Geometry: final body of the model. Coordinates: model frame, mm. Face numbers are marked on the shaded views. A direction names the side the tool comes from. Give positions to 0.01 mm unless a question says otherwise; leave off trailing zeros. Loops run counter-clockwise (first coordinate to the right, second up) from the corner with the lowest first, then second, coordinate; pieces in that order, holes last. Notation, with made-up numbers: (-9.75, 34.25) -> (30.25, 34.25) arc R19 cw to (30.25, 40.25) -> close; hole circle Ø11 at (31.25, 76.25). An arc over 180 degrees is marked (long way). Answer in a Markdown table with one row per item. Add a question column.
from build123d import *

# Parameters (mm, degrees)
SKETCH1_R               = 6
BOSS_EXTRUDE1_DEPTH     = 20
SKETCH2_R               = 2.25
CUT_EXTRUDE1_DEPTH      = 20
SKETCH4_R               = 1.5
CUT_EXTRUDE2_DEPTH      = 45
BOSS_EXTRUDE2_START     = 11
SKETCH5_W               = 15.288681569
SKETCH5_H               = 20
SKETCH5_R               = 1.5
BOSS_EXTRUDE2_DEPTH     = 11
CUT_EXTRUDE3_REACH      = 89.238
CUT_EXTRUDE3_END_RADIUS = 6
SKETCH6_R               = 1.25
SKETCH7_R               = 3
CUT_EXTRUDE4_DEPTH      = 5
CUT_EXTRUDE5_DEPTH      = 5
FILLET1_R               = 5
BOSS_EXTRUDE3_START     = 1
SKETCH10_R              = 3
SKETCH10_R_2            = 1.5
BOSS_EXTRUDE3_DEPTH     = 1
CHAMFER1_SIZE           = 1
SKETCH11_R              = 3
SKETCH11_R_2            = 1.5
BOSS_EXTRUDE4_DEPTH     = 1
CHAMFER2_SIZE           = 1


with BuildPart() as part:
    # Sketch1 → Boss-Extrude1 (new body)
    with BuildSketch(Plane.XY):
        Polygon((27, 30.8), (27, 25.8), (13, 25.8), (13, -7), (42, -7), (42, -13), (-7, -13), (-7, -43), (-13, -43), (-13, -8.291544952), (-13, 30.8), align=None)
        with Locations((0.051684878, 5)):
            Circle(SKETCH1_R, mode=Mode.SUBTRACT)
    extrude(amount=BOSS_EXTRUDE1_DEPTH)

    # Sketch2 → Cut-Extrude1 (cut)
    with BuildSketch(Plane.ZY.offset(13)):
        with Locations(Location((10, -38, 0), (0, 0, 270))):
            Circle(SKETCH2_R)
        with Locations(Location((10, -23, 0), (0, 0, 270))):
            Circle(SKETCH2_R)
    extrude(amount=-CUT_EXTRUDE1_DEPTH, mode=Mode.SUBTRACT)

    # Sketch4 → Cut-Extrude2 (cut)
    with BuildSketch(Plane(origin=(0, 30.8, 0), x_dir=(1, 0, 0), z_dir=(0, 1, 0))):
        with Locations(Location((22, -10, 0), (0, 0, 180))):
            Circle(SKETCH4_R)
        with Locations(Location((36, -10, 0), (0, 0, 180))):
            Circle(SKETCH4_R)
    extrude(amount=-CUT_EXTRUDE2_DEPTH, mode=Mode.SUBTRACT)

    # Sketch5 → Boss-Extrude2 (add)
    with BuildSketch(Plane(origin=(0, -7, 0), x_dir=(1, 0, 0), z_dir=(0, 1, 0)).offset(BOSS_EXTRUDE2_START)):
        with Locations((20.355659216, -10)):
            Rectangle(SKETCH5_W, SKETCH5_H)
        with Locations(Location((22, -10, 0), (0, 0, 180))):
            Circle(SKETCH5_R, mode=Mode.SUBTRACT)
    extrude(amount=-BOSS_EXTRUDE2_DEPTH)

    # Cut-Extrude3: up to this cylinder (the profile starts outside it)
    cut_extrude3_end = Plane(origin=(0.051684878, 5, 10), z_dir=(0, 0, -1)) * Cylinder(CUT_EXTRUDE3_END_RADIUS, 191.476, mode=Mode.PRIVATE)
    # Sketch6 → Cut-Extrude3 (cut, up to the surface)
    with BuildSketch(Plane(origin=(0, 30.8, 0), x_dir=(1, 0, 0), z_dir=(0, 1, 0)), mode=Mode.PRIVATE) as cut_extrude3_sk1:
        with Locations(Location((0, -10, 0), (0, 0, 180))):
            Circle(SKETCH6_R)
    cut_extrude3_tool1 = extrude(cut_extrude3_sk1.sketch, amount=-CUT_EXTRUDE3_REACH, mode=Mode.PRIVATE) - cut_extrude3_end
    add(cut_extrude3_tool1.solids().sort_by_distance((0, 30.8, 10))[0], mode=Mode.SUBTRACT)

    # Sketch7 → Cut-Extrude4 (cut)
    with BuildSketch(Plane(origin=(0, 30.8, 0), x_dir=(1, 0, 0), z_dir=(0, 1, 0))):
        with Locations(Location((0, -10, 0), (0, 0, 180))):
            Circle(SKETCH7_R)
    extrude(amount=-CUT_EXTRUDE4_DEPTH, mode=Mode.SUBTRACT)

    # Sketch9 → Cut-Extrude5 (cut)
    with BuildSketch(Plane.XZ.offset(13)):
        Polygon((25.233161507, 10), (23.616580754, 12.8), (20.383419246, 12.8), (18.766838493, 10), (20.383419246, 7.2), (23.616580754, 7.2), align=None)
    extrude(amount=-CUT_EXTRUDE5_DEPTH, mode=Mode.SUBTRACT)

    # Fillet1
    fillet1_edges = [part.edges().sort_by_distance(p)[0] for p in [
        (-13, 30.8, 10),
    ]]
    fillet(fillet1_edges, radius=FILLET1_R)

    # Sketch10 → Boss-Extrude3 (add)
    with BuildSketch(Plane(origin=(0, 4, 0), x_dir=(1, 0, 0), z_dir=(0, 1, 0)).offset(BOSS_EXTRUDE3_START)):
        with Locations(Location((22, -10, 0), (0, 0, 180))):
            Circle(SKETCH10_R)
        with Locations(Location((22, -10, 0), (0, 0, 180))):
            Circle(SKETCH10_R_2, mode=Mode.SUBTRACT)
    extrude(amount=-BOSS_EXTRUDE3_DEPTH)

    # Chamfer1
    chamfer1_edges = [part.edges().sort_by_distance(p)[0] for p in [
        (25, 5, 10),
    ]]
    chamfer(chamfer1_edges, length=CHAMFER1_SIZE - 0.0001)  # a hair under: the kernel refuses the full size

    # Sketch11 → Boss-Extrude4 (add)
    with BuildSketch(Plane.XZ.offset(-25.8)):
        with Locations(Location((22, 10, 0), (0, 0, 180))):
            Circle(SKETCH11_R)
        with Locations(Location((22, 10, 0), (0, 0, 180))):
            Circle(SKETCH11_R_2, mode=Mode.SUBTRACT)
    extrude(amount=BOSS_EXTRUDE4_DEPTH)

    # Chamfer2
    chamfer2_edges = [part.edges().sort_by_distance(p)[0] for p in [
        (25, 24.8, 10),
    ]]
    chamfer(chamfer2_edges, length=CHAMFER2_SIZE - 0.0001)  # a hair under: the kernel refuses the full size


solid = part.part
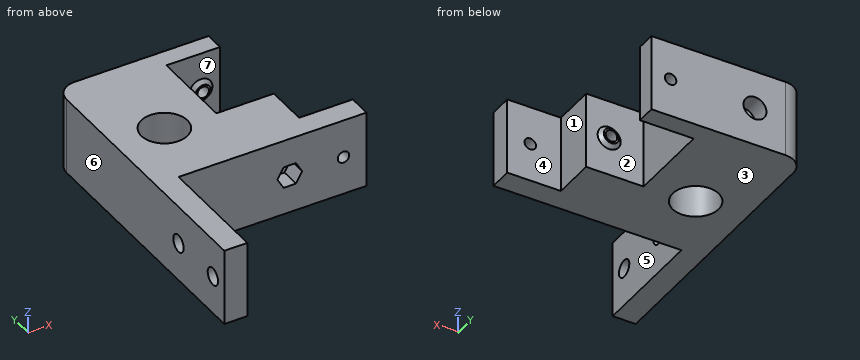
(1) Cut plane C-C on z = 16.5. Return the cut outline in (x, y), then the cut area to 3 significant figures.
(2) Cut plane B-B on y = -38. Return the cut outline in (x, z).
(3) Cut plane D-D on y = 20.5. Return the cut outline in (x, z).
(4) Cut plane A-A on x = 26. Return the cut outline in (y, z).
(5) Material intervals for line 1 along Z through (x, y) = (-11.4, -23); line 2 along Y through (x, z) = (22, 15); line 3 along Z through (x, y) = (36, -10.9), sorted ascending. Write a range as from..to.
(6) Reachability of the marked faces 4, 5, 6 and 7 from +Z, -Z, +X, -X, +Y, -Y: full face, straight path, thin tool, end or side. Return the list, or none.
(7) Pin query (flat end, axial travel): pin 1 Ø5 at (x, z) = (36, 10) entering from +Y; pin 2 Ø1.5 at (x, z) = (0, 10) entering from +Y; pin 3 Ø4 at (x, z) = (26.5, 14.5) entering from -Y; pin 4 Ø3.5 at (y, z) = (-38, 10) entering from -X. Return the tip coordinate at first contact, or that it passes through.
(8) Draft query along X for the marked faces 1, 2 and 3. Return one class per face: +X half, -X half, draft (parallel to the pull), parting line (faces both ways), or undercut.
Answer list:
| question | item | result |
|---|---|---|
| 1 | outline | (-13, -43) -> (-7, -43) -> (-7, -13) -> (42, -13) -> (42, -7) -> (28, -7) -> (28, 4) -> (13, 4) -> (13, 25.8) -> (27, 25.8) -> (27, 30.8) -> (-8, 30.8) arc R5 ccw to (-13, 25.8) -> close; hole circle Ø12 at (0.05, 5) |
| 1 | area | 1,610 mm² |
| 2 | outline | (-13, 0) -> (-7, 0) -> (-7, 7.75) -> (-13, 7.75) -> close; (-13, 12.25) -> (-7, 12.25) -> (-7, 20) -> (-13, 20) -> close |
| 3 | outline | (-13, 0) -> (13, 0) -> (13, 20) -> (-13, 20) -> close; hole circle Ø2.5 at (0, 10) |
| 4 | outline | (-13, 0) -> (4, 0) -> (4, 20) -> (-13, 20) -> close; (25.8, 0) -> (30.8, 0) -> (30.8, 20) -> (25.8, 20) -> close |
| 5 | line 1 | z = 0..7.75, 12.25..20 |
| 5 | line 2 | y = -13..4, 25.8..30.8 |
| 5 | line 3 | z = 0..8.5, 11.5..20 |
| 6 | face 4 | +Z, -Z, +X, +Y |
| 6 | face 5 | +Z, -Z, +X, -Y |
| 6 | face 6 | +Z, -Z, -X, +Y, -Y |
| 6 | face 7 | none |
| 7 | pin 1 | stops at y = -7 |
| 7 | pin 2 | stops at y = -0.95 |
| 7 | pin 3 | stops at y = -13 |
| 7 | pin 4 | passes through |
| 8 | face 1 | +X half |
| 8 | face 2 | undercut |
| 8 | face 3 | draft |
